```python
from build123d import *

# Parameters (mm, degrees)
SKETCH1_R               = 25.4
BOSS_EXTRUDE1_DEPTH     = 10.16
CUT_EXTRUDE2_DEPTH      = 12.16
CUT_EXTRUDE2_DEPTH_BACK = 12.16
SKETCH2_R               = 4.7625
CUT_EXTRUDE4_DEPTH      = 12.16
CUT_EXTRUDE4_DEPTH_BACK = 12.16
SKETCH3_W               = 3.175
SKETCH3_H               = 3.90525


with BuildPart() as part:
    # Sketch1 → Boss-Extrude1 (new body)
    with BuildSketch(Plane.XY):
        with Locations((0, -5.08)):
            Circle(SKETCH1_R)
    extrude(amount=BOSS_EXTRUDE1_DEPTH)

    # Sketch2 → Cut-Extrude2 (cut, two sides: drawn at the far end of the back side and taken through both)
    with BuildSketch(Plane.XY.offset(-CUT_EXTRUDE2_DEPTH_BACK)):
        Circle(SKETCH2_R)
    extrude(amount=CUT_EXTRUDE2_DEPTH + CUT_EXTRUDE2_DEPTH_BACK, mode=Mode.SUBTRACT)

    # Sketch3 → Cut-Extrude4 (cut, two sides: drawn at the far end of the back side and taken through both)
    with BuildSketch(Plane.XY.offset(-CUT_EXTRUDE4_DEPTH_BACK)):
        with Locations((0, 4.333875)):
            Rectangle(SKETCH3_W, SKETCH3_H)
    extrude(amount=CUT_EXTRUDE4_DEPTH + CUT_EXTRUDE4_DEPTH_BACK, mode=Mode.SUBTRACT)


solid = part.part
```
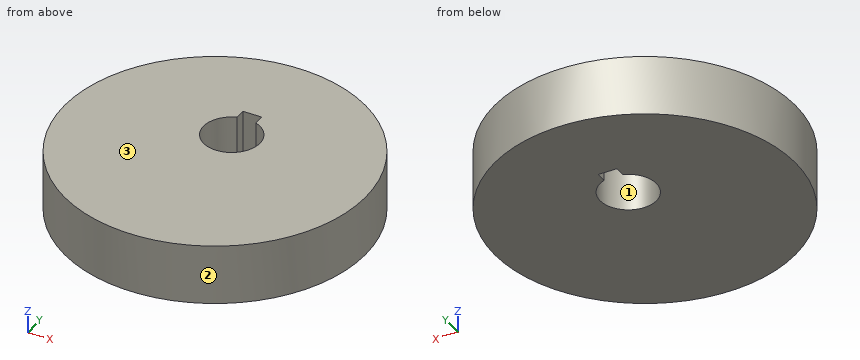
Source: CAD feature listing. Evaluate the final solid. Frame: model axes, mm. Face numbers are marked on the shaded views. Give positions to 0.01 mm unless a question says otherwise; leave off trailing zeros. Order: outer loops, then holes, each group sorted by start corner. A loop starts at its lowest first (then second) coordinate and runs counter-clockwise, first axis right, second up. Notation, with made-up numbers: (48, 87) -> (101, 87) arc R21 ccw to (101, 114) -> close; hole circle Ø9 at (35, -2.75). An arc over 180 degrees is marked (long way). Use a Markdown table: item, result.
Q1. Section B-B (z = 3.25). Return the cut outline in (x, y) (1 decimal), and give its area (3 significant figures).
A:
| item | result |
|---|---|
| outline | circle Ø50.8 at (0, -5.1); hole (-1.6, 4.5) arc R4.8 ccw (long way) to (1.6, 4.5) -> (1.6, 6.3) -> (-1.6, 6.3) -> close |
| area | 1,950 mm^2 |
Q2. Section D-D (y = -26). Return the cut outline in (x, z).
A:
| item | result |
|---|---|
| outline | (-14.41, 0) -> (14.41, 0) -> (14.41, 10.16) -> (-14.41, 10.16) -> close |
Q3. First-contact query: P1, Ø1.4, axis at y = 5, z = 7.5, coming from the -X side; P2, Ø4, axis at y = -20.5, z = 4, coming from the -X side; P3, Ø0.9, axis at y = 5.5, z = 5, coming from the +X side. Flat tips, straight axial feed; report the tip coordinate or a pass-through.
A:
| item | result |
|---|---|
| P1 | x = -23.6 |
| P2 | x = -21.57 |
| P3 | x = 23.29 |
Q4. Material intervals for line 1 (Y direction, x = 0, z = 5.25); line 2 (X direction, y = 0, z = 6.75); line 3 (X direction, y = 6, z = 8.25), sorted ascending. Write a range as [from, to].
A:
| item | result |
|---|---|
| line 1 | [-30.48, -4.76], [6.29, 20.32] |
| line 2 | [-24.89, -4.76], [4.76, 24.89] |
| line 3 | [-22.86, -1.59], [1.59, 22.86] |
Q5. Section A-A (x = 0). Return the cut outline in (y, z), and give its area (3 significant figures).
A:
| item | result |
|---|---|
| outline | (-30.48, 0) -> (-4.76, 0) -> (-4.76, 10.16) -> (-30.48, 10.16) -> close; (6.29, 0) -> (20.32, 0) -> (20.32, 10.16) -> (6.29, 10.16) -> close |
| area | 404 mm^2 |
Q6. Pull-direction query (Y, two-part tool) for the marked faces 1, 2 and 3; classes: +Y half, -Y half, draft (parallel to the pull), parting line (faces both ways), or undercut.
A:
| item | result |
|---|---|
| face 1 | undercut |
| face 2 | parting line |
| face 3 | draft |
Q7. Section C-C (y = 1). Return the cut outline in (x, z).
A:
| item | result |
|---|---|
| outline | (-24.66, 0) -> (-4.66, 0) -> (-4.66, 10.16) -> (-24.66, 10.16) -> close; (4.66, 0) -> (24.66, 0) -> (24.66, 10.16) -> (4.66, 10.16) -> close |
